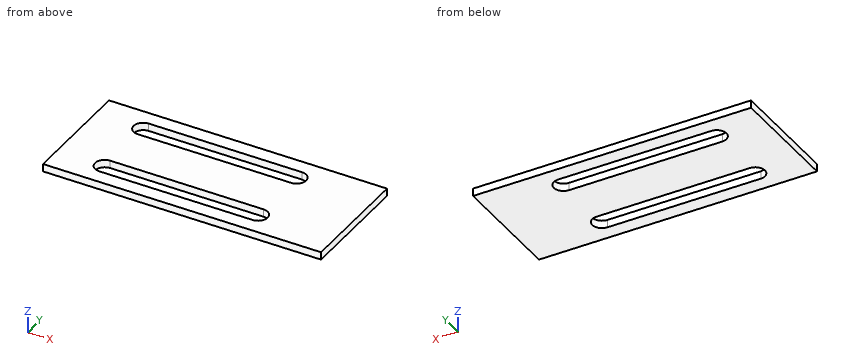
Autodesk Inventor part; units mm, degrees
ref_plane "YZ Plane" through (0, 0, 0) normal (1, 0, 0) x (0, 1, 0)
ref_plane "XZ Plane" through (0, 0, 0) normal (0, 1, 0) x (-1, 0, 0)
ref_plane "XY Plane" through (0, 0, 0) normal (0, 0, 1) x (1, 0, 0)
sketch "Sketch3" plane through (0, 0, 0) normal (0, 0, 1) x (1, 0, 0)
  line L0 (-101.5, 0) -> (101.5, 0)
  line L1 (0, -42) -> (0, 42)
  line L2 (-72.5, -30) -> (72.5, -30)
  line L3 (72.5, -30) -> (72.5, 30)
  line L4 (72.5, 30) -> (-72.5, 30)
  line L5 (-72.5, 30) -> (-72.5, -30)
  line L6 (-72.5, -30) -> (72.5, 30) construction
  line L7 (72.5, -30) -> (-72.5, 30) construction
  line L8 (-47.5, 17.5) -> (32.5, 17.5) construction
  line L9 (-47.5, 12.5) -> (32.5, 12.5)
  line L10 (32.5, 22.5) -> (-47.5, 22.5)
  arc A0 (-47.5, 22.5) -> (-47.5, 12.5) centre (-47.5, 17.5) ccw
  arc A1 (32.5, 12.5) -> (32.5, 22.5) centre (32.5, 17.5) ccw
  line L11 (-49.3038, -17.5) -> (32.5, -17.5) construction
  line L12 (-47.5, -22.5) -> (32.5, -22.5)
  line L13 (32.5, -12.5) -> (-47.5, -12.5)
  arc A2 (-47.5, -12.5) -> (-47.5, -22.5) centre (-47.5, -17.5) ccw
  arc A3 (32.5, -22.5) -> (32.5, -12.5) centre (32.5, -17.5) ccw
  point P0 (0, 0)
  dimension "d0" = 145
  dimension "d1" = 60
  dimension "d2" = 10
  dimension "d3" = 10
  dimension "d4" = 35
  dimension "d9" = 32.5
  dimension "d10" = 32.5
  dimension "d11" = 47.5
  dimension "d12" = 47.5
extrude "Extrusion1" add sketch "Sketch3" along normal blind 4 contours L5 L4 L1 L10 A0 L9 L0 | L0 L1 L13 A2 L12 L2 L5 | L1 L9 A1 L10 L4 L3 L0 | L0 L3 L2 L1 L12 A3 L13
equation "\"d3\" = d2"
equation "\"d10\" = d9"
equation "\"d12\" = d11"
equation "\"BendRadius\" = Thickness"
equation "\"BendReliefWidth\" = Thickness"
equation "\"BendReliefDepth\" = 0.5 * Thickness"
equation "\"CornerReliefSize\" = 4 * Thickness"
equation "\"MinimumRemnant\" = 2 * Thickness"
equation "\"TransitionRadius\" = BendRadius"
equation "\"JacobiRadiusSize\" = BendRadius"
equation "\"GapSize\" = Thickness"
properties part number "Motor holder slider"
Geometry check sheet. Reference: the model listing, model coordinates, mm. Round coordinates to 2 decimals unless told otherwise and drop trailing zeros. Order: outer loops, then holes, each group sorted by start corner. A loop starts at its lowest first (then second) coordinate and runs counter-clockwise, first axis right, second up. Notation, with made-up numbers: M -35.75,-2.75 L -8.75,-2.75 A25 cw -8.75,21.25 Z; hole C 8,50.25 d6. An arc over 180 degrees is marked long. Write item = value, one per line.
Q1. Section check B-B (y = 17.5). Enter the section's corners in (x, z), plus the area to 3 significant figures.
Answer block:
outline = M -72.5,0 L -52.5,0 L -52.5,4 L -72.5,4 Z; M 37.5,0 L 72.5,0 L 72.5,4 L 37.5,4 Z
area = 220 mm^2
Q2. Scan lines: line 1 (Y direction, x = -45, z = 1.8); line 2 (X direction, y = -20.5, z = 3.7). Record each from-to range of solid material in increasing order.
Answer block:
line_1 = -30 to -22.5, -12.5 to 12.5, 22.5 to 30
line_2 = -72.5 to -51.5, 36.5 to 72.5
Q3. Section check A-A (x = -46). Enter the section's corners in (y, z), plus the area to 3 significant figures.
Answer block:
outline = M -30,0 L -22.5,0 L -22.5,4 L -30,4 Z; M -12.5,0 L 12.5,0 L 12.5,4 L -12.5,4 Z; M 22.5,0 L 30,0 L 30,4 L 22.5,4 Z
area = 160 mm^2
